Design review of the part shown in the three views and the two pictorial views. Dimensions are in mm from the part's minimum x, y and z. A direction names the side the tool comes from. Round coordinates to 2 decimals unless told otherwise and drop trailing zeros. Loops run counter-clockwise (first coordinate to the right, second up) from the corner with the lowest first, then second, coordinate; pieces in that order, holes last. Notation, with made-up numbers: (-24.5, -37.75) -> (-7.5, -37.75) arc R17 cw to (-7.5, -13.75) -> close; hole circle Ø8 at (50.25, 47). An arc over 180 degrees is marked (long way). One line per question, with ' | ' between items. Start each with the question number.
1. Consider section C-C (z = 7.75). Write out the cut boundary in (x, y), and give its area (3 significant figures).
2. For the marked faces 5 and 6, list the 3-axis set-ups (+Z, -Z, +X, -X, +Y, -Y) from which the entire face can be reached by the end or side of a thin tool; tool diameter is ignored.
3. For pin 1 Ø12 at (x, y) = (20, 15) entering from +Z; pin 2 Ø1 at (x, y) = (23, 25.5) entering from -Z, all flat-tipped, find the tip position at first contact; note any pin that passes through.
4. Consider section D-D (y = 4.5). Write out the cut boundary in (x, z).
5. Consider section A-A (y = 15). Write out the cut boundary in (x, z).
6. Wall thickness on line 1 along Y through (x, z) = (20, 12.15); line 2 along X through (y, z) = (5, 5.5); line 3 along X through (y, z) = (10.75, 11.5): over which ranges is each line inside the solid? List them lowest first.
7. Consider section B-B (x = 20). Write out the cut boundary in (y, z).
8. Draft analysis for pull direction X (two halves, no side actions). For the marked faces 1, 2, 3 and 4, state which applies: pulls with the +X half, pulls with the -X half, needs draft (parallel to the pull), parting line crosses it, or undercut.
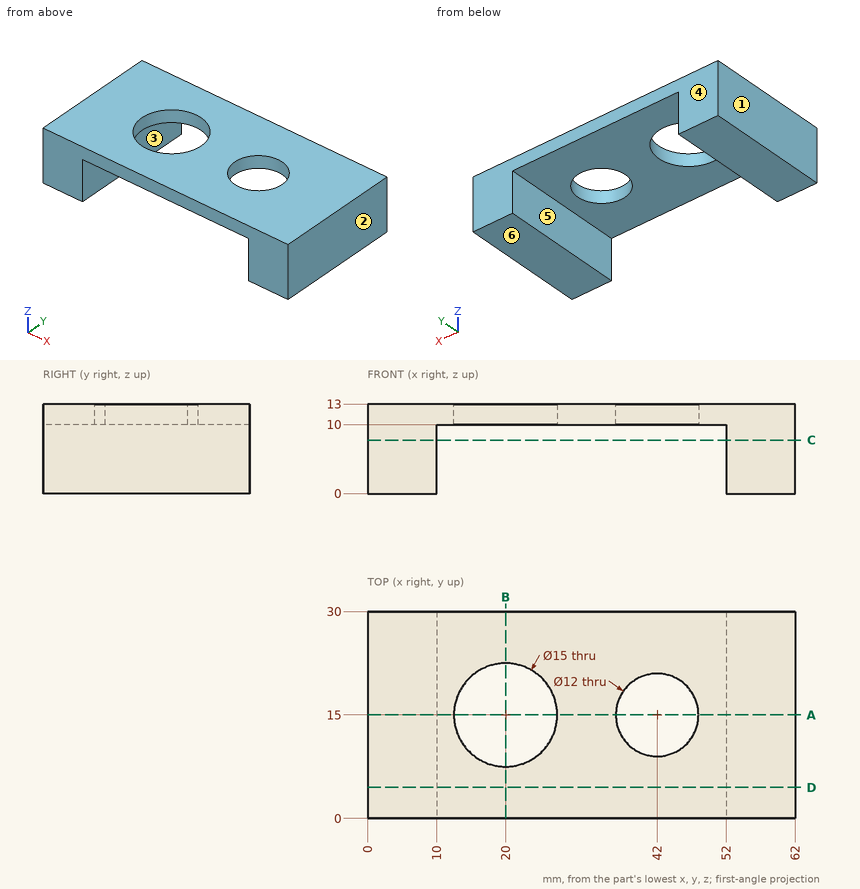
Answer block:
1) outline: (0, 0) -> (10, 0) -> (10, 30) -> (0, 30) -> close; (52, 0) -> (62, 0) -> (62, 30) -> (52, 30) -> close | area: 600 mm2
2) face 5: -Z, +Y, -Y | face 6: -Z, +X, -X, +Y, -Y
3) pin 1: passes through | pin 2: stops at z = 10
4) outline: (0, 0) -> (10, 0) -> (10, 10) -> (52, 10) -> (52, 0) -> (62, 0) -> (62, 13) -> (0, 13) -> close
5) outline: (0, 0) -> (10, 0) -> (10, 10) -> (12.5, 10) -> (12.5, 13) -> (0, 13) -> close; (27.5, 10) -> (36, 10) -> (36, 13) -> (27.5, 13) -> close; (48, 10) -> (52, 10) -> (52, 0) -> (62, 0) -> (62, 13) -> (48, 13) -> close
6) line 1: y = 0 to 7.5, 22.5 to 30 | line 2: x = 0 to 10, 52 to 62 | line 3: x = 0 to 13.82, 26.18 to 37.76, 46.24 to 62
7) outline: (0, 10) -> (7.5, 10) -> (7.5, 13) -> (0, 13) -> close; (22.5, 10) -> (30, 10) -> (30, 13) -> (22.5, 13) -> close
8) face 1: pulls with the -X half | face 2: pulls with the +X half | face 3: undercut | face 4: needs draft
